Part model, mm, in its own coordinate system. A direction names the side the tool comes from. Give positions to 0.01 mm unless a question says otherwise; leave off trailing zeros. Order: outer loops, then holes, each group sorted by start corner. A loop starts at its lowest first (then second) coordinate and runs counter-clockwise, first axis right, second up. Notation, with made-up numbers: (13.5, 4) - (45.5, 4) arc R13 ccw to (45.5, 29) - close; hole circle Ø5 at (72, 87). An arc over 180 degrees is marked (long way). One line per item, written item: value.
```python
from build123d import *

# Parameters (mm, degrees)
F0_R     = 28.575
F1_DEPTH = 3.175
F3_DEPTH = 3.176


# Not quite as in the source:
# - a length typed as a fraction of an inch, garbled in the dataset ("3 / 203.2 mm" for 3/8 in), is restored


with BuildPart() as f1:
    # F0 (on Front) → F1 (new body)
    with BuildSketch(Plane.XZ):
        Circle(F0_R)
    extrude(amount=F1_DEPTH)

    # F2 (on face) → F3 (cut, through all)
    with BuildSketch(Plane.XZ.offset(3.175)):
        with BuildLine():
            Line((7.2536082684, 0), (0, 0))
            Line((0, 0), (0, -19.575))
            ThreePointArc((0, -19.575), (5.3192801015, -10.4146549257), (7.2536082684, 0))
        make_face()
        with BuildLine():
            Line((0, -19.575), (0, 0))
            Line((0, 0), (-6.9936556862, 0))
            ThreePointArc((-6.9936556862, 0), (-5.0483188999, -10.341808774), (0, -19.575))
        make_face()
        with BuildLine():
            ThreePointArc((-6, 9.1323722154), (-6.8103344804, 4.6002974695), (-6.9936556862, 0))
            Line((-6.9936556862, 0), (0, 0))
            Line((0, 0), (7.2536082684, 0))
            ThreePointArc((7.2536082684, 0), (6.9672213091, 4.6129154541), (6, 9.1323722154))
            Line((6, 9.1323722154), (6, 18.5192639611))
            Line((6, 18.5192639611), (9.3, 18.5192639611))
            Line((9.3, 18.5192639611), (9.3, 27.0192639611))
            ThreePointArc((9.3, 27.0192639611), (0, 28.575), (-9.3, 27.0192639611))
            Line((-9.3, 27.0192639611), (-9.3, 18.5192639611))
            Line((-9.3, 18.5192639611), (-6, 18.5192639611))
            Line((-6, 18.5192639611), (-6, 9.1323722154))
        make_face()
        with BuildLine():
            ThreePointArc((-16.0375, -23.650142045), (-14.3234197578, -24.7259028438), (-12.5375, -25.6776501797))
            Line((-12.5375, -25.6776501797), (-12.5375, 0))
            Line((-12.5375, 0), (-16.0375, 0))
            Line((-16.0375, 0), (-16.0375, -23.650142045))
        make_face()
        with BuildLine():
            Line((-1.75, -24.075), (-1.75, -28.5213626077))
            ThreePointArc((-1.75, -28.5213626077), (-0.8754108992, -28.5615875042), (0, -28.575))
            Line((0, -28.575), (0, -24.075))
            Line((0, -24.075), (-1.75, -24.075))
        make_face()
        with BuildLine():
            Line((0, -24.075), (0, -28.575))
            ThreePointArc((0, -28.575), (0.8754108992, -28.5615875042), (1.75, -28.5213626077))
            Line((1.75, -28.5213626077), (1.75, -24.075))
            Line((1.75, -24.075), (0, -24.075))
        make_face()
        with BuildLine():
            Line((12.5375, 0), (12.5375, -25.6776501797))
            ThreePointArc((12.5375, -25.6776501797), (14.3234197578, -24.7259028438), (16.0375, -23.650142045))
            Line((16.0375, -23.650142045), (16.0375, 0))
            Line((16.0375, 0), (12.5375, 0))
        make_face()
    extrude(amount=-F3_DEPTH, mode=Mode.SUBTRACT)


solid = f1.part
```
1) Which spindle directions (+Z, -Z, +X, -X, +Y, -Y) get a long thin tool onto all of the face, cutting with end or side? Do faces 1 (the face through (-6, -2, 14)), 2 (the face through (7.21, -1.57, -27.65)), 3 (the face through (14, -2, 0)). Say none if no direction does.
Answer:
face 1: +Z, +Y, -Y
face 2: -Z, +X, +Y, -Y
face 3: -Z, +Y, -Y
2) Wall check: line 1 along X through (y, z) = (-1.75, -3.5); line 2 along X through (y, z) = (-0.2, -21); line 3 along X through (y, z) = (-0.7, -15.5). Give the ranges that are in metal, low to high. Write a range as [from, to].
Answer:
line 1: x = [-28.36, -16.04], [-12.54, -6.71], [7.01, 12.54], [16.04, 28.36]
line 2: x = [-19.38, -16.04], [-12.54, 12.54], [16.04, 19.38]
line 3: x = [-24.01, -16.04], [-12.54, -2.7], [2.89, 12.54], [16.04, 24.01]
3) Drop flat-ended pins along their axis: P1, Ø1, axis at y = -2, z = -9, coming from the +X side; P2, Ø1.6, axis at y = -1, z = 21, coming from the +X side; P3, Ø1.6, axis at y = -1, z = 13.5, coming from the +X side; P4, Ø12, axis at x = 9, z = -23, coming from the +Y side. Give the stop position or say it passes through.
Answer:
P1: stops at x = 27.28
P2: stops at x = 20.21
P3: stops at x = 25.6
P4: stops at y = 0
4) Two-plate mould, pull along X, no slides. Class faces 4 (the face through (-28.264, -1.565, 4.205)), 5 (the face through (6, -2, 14)), 6 (the face through (28.38, -1.57, 3.33)): pulls with the +X half, pulls with the -X half, needs draft (parallel to the pull), parting line crosses it, or undercut.
Answer:
face 4: pulls with the -X half
face 5: undercut
face 6: pulls with the +X half
5) Slice it at C-C on z = -13. Write the cut outline in (x, y) (1 decimal).
Answer:
outline: (-25.4, -3.2) - (-16, -3.2) - (-16, 0) - (-25.4, 0) - close; (-12.5, -3.2) - (-4, -3.2) - (-4, 0) - (-12.5, 0) - close; (4.2, -3.2) - (12.5, -3.2) - (12.5, 0) - (4.2, 0) - close; (16, -3.2) - (25.4, -3.2) - (25.4, 0) - (16, 0) - close
6) Slice it at A-A on z = 5.5. Write the cut outline in (x, y) (3 decimals), then the cut area to 3 significant figures.
Answer:
outline: (-28.041, -3.175) - (-6.7, -3.175) - (-6.7, 0) - (-28.041, 0) - close; (6.832, -3.175) - (28.041, -3.175) - (28.041, 0) - (6.832, 0) - close
area: 135 mm2
7) Slice it at D-D on x = 19. Write the cut outline in (y, z) (3 decimals).
Answer:
outline: (-3.175, -21.343) - (0, -21.343) - (0, 21.343) - (-3.175, 21.343) - close
